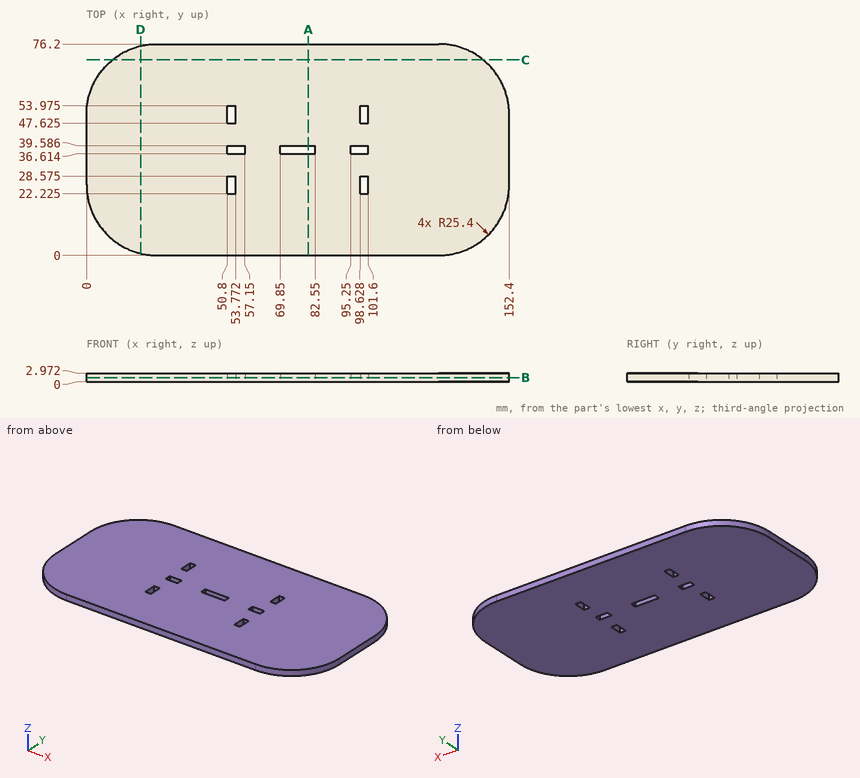
The figure shows three views and two pictorial views of one solid part (mm, origin at its lowest corner). Answer the questions. Coordinates: 2 decimals unless noted, no trailing zeros. Loops run counter-clockwise (first coordinate to the right, second up) from the corner with the lowest first, then second, coordinate; pieces in that order, holes last.
1) Find section D-D on x = 19.5. Write down the section's boundary in (y, z) (1 decimal), then the cut area to 3 significant figures.
2) Find section B-B on z = 1.45. Give the number of separate pieces and of enclosed holes in the cut face, then the cut area to 3 significant figures.
3) Find section A-A on x = 80. Write down the section's boundary in (y, z), then the cut area to 3 significant figures.
4) Find section C-C on y = 70.5. Write down the section's boundary in (x, z), then the cut area to 3 significant figures.
5) A flat-ended cylindrical pin translates along its axis: pin 1 Ø1.5 at (y, z) = (54.5, 1.5) entering from -X. Find the tip coordinate at first contact, or state that the pin passes through.
6) Find the intervals of material crossed by L1, parallel to X at y = 28, z = 1.95; L2, parallel to X at y = 37, z = 2.4; L3, parallel to X at y = 53.5, z = 2.85, in increasing order.
Values:
1. outline: (0.7, 0) - (75.5, 0) - (75.5, 3) - (0.7, 3) - close
1. area: 222 mm2
2. separate pieces: 1
2. enclosed holes: 7
2. area: 10,900 mm2
3. outline: (0, 0) - (36.61, 0) - (36.61, 2.97) - (0, 2.97) - close; (39.59, 0) - (76.2, 0) - (76.2, 2.97) - (39.59, 2.97) - close
3. area: 218 mm2
4. outline: (9.37, 0) - (143.03, 0) - (143.03, 2.97) - (9.37, 2.97) - close
4. area: 397 mm2
5. pin 1: stops at x = 0.17
6. L1: x = 0 to 50.8, 53.77 to 98.63, 101.6 to 152.4
6. L2: x = 0 to 50.8, 57.15 to 69.85, 82.55 to 95.25, 101.6 to 152.4
6. L3: x = 0.14 to 50.8, 53.77 to 98.63, 101.6 to 152.26
